For this review, take the finished solid that the model builds, in its own axes (mm). A direction names the side the tool comes from. Round coordinates to 2 decimals unless told otherwise and drop trailing zeros. Write each loop counter-clockwise with the first axis right and the second up, starting at its lowest first coordinate (ties: lowest second). Pieces come first, ordered by that corner, then holes. Notation, with made-up numbers: M 75,41 L 114,41 A20 ccw 114,73 Z; hole C 33,-31 d8. An arc over 180 degrees is marked long. Use one line per item in the form item = value. Start each with the question number.
Item 1: For line 1 (X direction, y = 4.55, z = 0); line 2 (Y direction, x = 3.5, z = 6.5), list the stretches that pass through material, from the lowest coordinate up. Write a range as [from, to].
Item 2: Add section B-B (z = -5). State the section outline as (x, y) points, and give its area (3 significant figures).
Item 3: For P1, Ø0.7, axis at x = 6.5, y = -1, coming from the +Z side; P2, Ø2, axis at x = 3.5, y = -2.5, coming from the -Z side, all flat-tipped, find the tip position at first contact; note any pin that passes through.
Item 4: For faces 1 (the cylindrical face through (-1.27, -4.49, 0.97)), 2 (the flat face through (0, 4, 2)), 3 (the flat face through (-7, 0, 0)), list the 3-axis set-ups (+Z, -Z, +X, -X, +Y, -Y) from which the entire face can be reached by the end or side of a thin tool; tool diameter is ignored.
Item 5: Draft analysis for pull direction Y (two halves, no side actions). For faces 4 (the flat face through (0, -5, 2)), 5 (the cylindrical face through (0.976, -0.07, -7.436)), 6 (the flat face through (0, 5, 2)), 7 (the flat face through (7, 0, 0)), state which applies: released by +Y, released by -Y, zero draft, split by the parting line, or undercut.
Item 6: Add section C-C (z = 1.25). State the section outline as (x, y) points, and give its area (3 significant figures).
Item 7: Add section D-D (y = -1.25). State the section outline as (x, z) points, and give its area (3 significant figures).
Item 8: Add section A-A (x = 0). State the section outline as (y, z) points.
Autodesk Inventor part; units mm, degrees
ref_plane "YZ Plane" through (0, 0, 0) normal (1, 0, 0) x (0, 1, 0)
ref_plane "XZ Plane" through (0, 0, 0) normal (0, 1, 0) x (-1, 0, 0)
ref_plane "XY Plane" through (0, 0, 0) normal (0, 0, 1) x (1, 0, 0)
sketch "Boceto1" plane through (0, 0, 0) normal (0, 1, 0) x (-1, 0, 0)
  circle A0 centre (0, 0) radius 7.5
  dimension "d0" = 15
extrude "Extrusión1" add sketch "Boceto1" along normal mid plane 10
sketch "Boceto2" plane through (0, 0, 0) normal (0, 1, 0) x (-1, 0, 0)
  circle A0 centre (0, 0) radius 6.15
  dimension "d3" = 12.3
extrude "Extrusión2" cut sketch "Boceto2" along normal mid plane 8
sketch "Boceto3" plane through (0, 5, 0) normal (0, 1, 0) x (1, 0, 0)
  circle A0 centre (0, 0) radius 1.6
  dimension "d6" = 3.2
extrude "Extrusión3" cut sketch "Boceto3" against normal through all
sketch "Boceto4" plane through (0, 0, 0) normal (0, 0, 1) x (1, 0, 0)
  line L0 (-10.1106, -4) -> (10.1106, -4)
  line L1 (10.1106, -4) -> (10.1106, 4)
  line L2 (10.1106, 4) -> (-10.1106, 4)
  line L3 (-10.1106, 4) -> (-10.1106, -4)
  line L4 (-10.1106, -4) -> (10.1106, 4) construction
  line L5 (10.1106, -4) -> (-10.1106, 4) construction
  line L6 (-7.5, -5) -> (7.5, -5)
  point P0 (0, 0)
  dimension "d11" = 8
  dimension "d12" = 1
extrude "Extrusión4" cut sketch "Boceto4" along normal through all
properties part number "Rubberfoot"
Calculated:
q1.line_1 = [-7.5, -1.6], [1.6, 7.5]
q1.line_2 = [-5, -4], [4, 5]
q2.outline = M -5.59,-5 L 5.59,-5 L 5.59,5 L -5.59,5 Z; hole M -3.58,-4 L 3.58,-4 L 3.58,4 L -3.58,4 Z
q2.area = 54.5 mm^2
q3.P1 = 0
q3.P2 = -7.07
q4.face_1 = +Y, -Y
q4.face_2 = +Z
q4.face_3 = +Z, +X, -X
q5.face_4 = released by -Y
q5.face_5 = zero draft
q5.face_6 = released by +Y
q5.face_7 = undercut
q6.outline = M -7.4,-5 L -1,-5 L -1,-4 L -7.4,-4 Z; M -7.4,4 L -1,4 L -1,5 L -7.4,5 Z; M 1,-5 L 7.4,-5 L 7.4,-4 L 1,-4 Z; M 1,4 L 7.4,4 L 7.4,5 L 1,5 Z
q6.area = 25.6 mm^2
q7.outline = M -7.5,0 A7.5 ccw 7.5,0 L 6.15,0 A6.15 cw -6.15,0 Z
q7.area = 28.9 mm^2
q8.outline = M -5,-7.5 L 5,-7.5 L 5,-1.6 L 4,-1.6 L 4,-6.15 L -4,-6.15 L -4,-1.6 L -5,-1.6 Z; M -5,1.6 L -4,1.6 L -4,7.5 L -5,7.5 Z; M 4,1.6 L 5,1.6 L 5,7.5 L 4,7.5 Z
